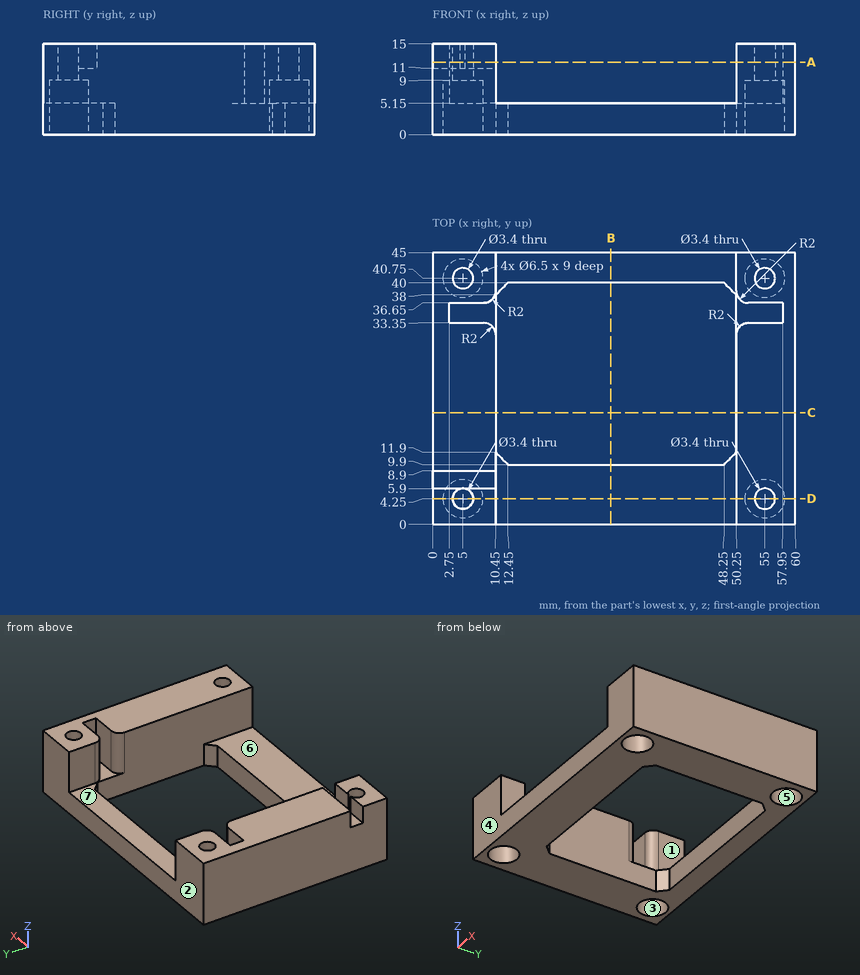
For this review, use the dimensioned drawing (mm, ordinates from the lowest corner) and the shaded views. A direction names the side the tool comes from. Round coordinates to 2 decimals unless told otherwise and drop trailing zeros. Write each loop counter-clockwise with the first axis right and the second up, starting at its lowest first coordinate (ties: lowest second). Pieces come first, ordered by that corner, then holes. Notation, with made-up numbers: (29.5, -20.75) - (38.5, -20.75) arc R33 ccw to (38.5, 12.25) - close; hole circle Ø9 at (21, 34.5). An arc over 180 degrees is marked (long way). Answer as CSV lines item,"result". Start each with the question number.
(1) For the marked faces 5, 6 and 7, list the 3-axis set-ups (+Z, -Z, +X, -X, +Y, -Y) from which the entire face can be reached by the end or side of a thin tool; tool diameter is ignored.
(2) To check wall thickness, follow line 1 (Y direction, x = 5, z = 2.5); line 2 (Y direction, x = 55, z = 7.25); line 3 (Y direction, x = 55, z = 11.1). State the ranges of each line that lie inside material, in increasing order.
(3) We need section B-B on x = 29.5. State the section outline as (y, z) points.
(4) Draft analysis for pull direction Y (two halves, no side actions). For the marked faces 1, 2, 3 and 4, state which applies: pulls with the +Y half, pulls with the -Y half, needs draft (parallel to the pull), parting line crosses it, or undercut.
(5) We need section C-C on y = 18.5. State the section outline as (x, z) points.
(6) We need section D-D on y = 4.25. State the section outline as (x, z) points, plus the area to 3 significant figures.
(7) We need section A-A on z = 12. Give the number of separate pieces and of enclosed holes in the cut face, plus the area to 3 significant figures.
(8) For pin 1 Ø2.5 at (x, y) = (4.5, 7.5) entering from +Z; pin 2 Ø4 at (x, y) = (29.5, 41.5) entering from +Z, all flat-tipped, find the tip position at first contact; note any pin that passes through.
Worked answers:
1,face 5,"-Z"
1,face 6,"+Z, +Y, -Y"
1,face 7,"+Z"
2,line 1,"0 to 1, 7.5 to 37.5, 44 to 45"
2,line 2,"0 to 1, 7.5 to 33.35, 36.65 to 37.5, 44 to 45"
2,line 3,"0 to 2.55, 5.95 to 33.35, 36.65 to 39.05, 42.45 to 45"
3,outline,"(0, 0) - (9.9, 0) - (9.9, 5.15) - (0, 5.15) - close; (40, 0) - (45, 0) - (45, 5.15) - (40, 5.15) - close"
4,face 1,"needs draft"
4,face 2,"pulls with the +Y half"
4,face 3,"undercut"
4,face 4,"pulls with the -Y half"
5,outline,"(0, 0) - (10.45, 0) - (10.45, 15) - (0, 15) - close; (50.25, 0) - (60, 0) - (60, 15) - (50.25, 15) - close"
6,outline,"(0, 0) - (1.75, 0) - (1.75, 9) - (3.3, 9) - (3.3, 15) - (0, 15) - close; (6.7, 9) - (8.25, 9) - (8.25, 0) - (51.75, 0) - (51.75, 9) - (53.3, 9) - (53.3, 15) - (50.25, 15) - (50.25, 5.15) - (10.45, 5.15) - (10.45, 15) - (6.7, 15) - close; (56.7, 9) - (58.25, 9) - (58.25, 0) - (60, 0) - (60, 15) - (56.7, 15) - close"
6,area,"350 mm²"
7,separate pieces,"3"
7,enclosed holes,"3"
7,area,"787 mm²"
8,pin 1,"z = 11"
8,pin 2,"z = 5.15"
